Input: part model. Units: mm. Frame: model coordinates. Give positions to 0.01 mm unless a question says otherwise; leave off trailing zeros. Loops run counter-clockwise (first coordinate to the right, second up) from the corner with the lowest first, then second, coordinate; pieces in that order, holes last. Notation, with made-up numbers: M -29,79.25 L -11,79.25 A16 ccw -11,95.25 Z; hole C 14.25,-30.75 d11. An arc over 180 degrees is marked long. Return JSON: item names as keys, results as strings. Group by question number.
```python
from build123d import *

# Parameters (mm, degrees)
F1_DEPTH = 100
F2_SIZE  = 4.99999


# Not quite as in the source:
# - a fillet or chamfer is up to 0.001 mm smaller than in the source, because OpenCascade refuses the exact size


with BuildPart() as f1:
    # F0 (on Right) → F1 (new body)
    with BuildSketch(Plane.YZ):
        Polygon((7.4991378996, -1.2852627068), (-4.5274403009, 10.7413154936), (-8.0629742068, 7.2057815877), (3.9636039936, -4.8207966127), align=None)
    extrude(amount=F1_DEPTH)

    # F2 (size 5 in the source; OpenCascade refuses exactly that, so slightly less here)
    f2_edges = [f1.edges().sort_by_distance(p)[0] for p in [
        (50, -8.062974, 7.205782),
        (50, 3.963604, -4.820797),
    ]]
    chamfer(f2_edges, length=F2_SIZE)


solid = f1.part
```
Item 1: First-contact query: pin 1 Ø3 at (x, y) = (36, 2) entering from +Z; pin 2 Ø1 at (y, z) = (5.5, 2) entering from +X; pin 3 Ø1 at (x, z) = (43.5, 2.5) entering from +Y; pin 4 Ø3 at (x, z) = (87, 4.5) entering from +Y. Flat tips, straight axial feed; report the tip coordinate or a pass-through.
Item 2: Section C-C, the plane z = 7.75. Return loops of the section in (x, y).
Item 3: Material intervals for line 1 (Z direction, x = 13.5, y = -1.5); line 2 (Z direction, x = 81.5, y = -4); line 3 (Y direction, x = 52, z = 3.75), sorted ascending. Write a range as from..to.
Item 4: Section B-B, the plane y = 4.5. Return loops of the section in (x, z), then the cut area to 3 significant figures.
Answer below:
{
 "1": {"pin 1": "z = 5.71", "pin 2": "through", "pin 3": "y = 4.21", "pin 4": "y = 3.21"},
 "2": {"outline": "M 0,-4.53 L 100,-4.53 L 100,-1.54 L 0,-1.54 Z"},
 "3": {"line 1": "0.64..7.71", "line 2": "3.14..10.21", "line 3": "-4.53..2.46"},
 "4": {"outline": "M 0,-1.29 L 100,-1.29 L 100,1.71 L 0,1.71 Z", "area": "300 mm^2"}
}
